Could you check a few things on this model? Use its own coordinates, in mm. Give positions to 0.01 mm unless a question says otherwise; leave off trailing zeros. Order: outer loops, then holes, each group sorted by start corner. A loop starts at its lowest first (then second) coordinate and runs counter-clockwise, first axis right, second up. Notation, with made-up numbers: (33.5, 47) -> (47.5, 47) arc R30 ccw to (47.5, 69) -> close; hole circle Ø5 at (68.25, 62.25). An arc over 180 degrees is marked (long way). Answer as CSV lines item,"result". Start each with the question number.
(1) Will this pin go through, and if not, where does the flat tip stop? pin 1 Ø1.5 at (x, z) = (-5.5, 0.5) entering from -Y.
(2) I want a section at C-C (x = 10.5). Please give me the cut outline in (y, z), plus the area to 3 significant figures.
(3) We'd pull the mould along Y, two halves only. Please class faces 1 (the face through (11.594, 2.281, 1.521)), 2 (the face through (2, 29, 3)), 3 (the face through (10.066, 26.548, 1.479)), 4 (the face through (11.719, 54.594, 1.521)): released by +Y, released by -Y, zero draft, split by the parting line, or undercut.
(4) I want a section at A-A (y = 28.5). Please give me the cut outline in (x, z), plus the area to 3 significant figures.
(5) I need wall thicknesses on L1, parallel to X at y = 28.5, z = 2.3; L2, parallel to Y at x = 10.5, z = 1.6; L3, parallel to Y at x = 9.5, z = 2.75. Which ranges of each line are inside material? Lowest first, please.
(6) I want a section at B-B (z = 1.05). Please give me the cut outline in (x, y).
(7) I want a section at D-D (y = 4.5). Please give me the cut outline in (x, z).
```python
from build123d import *

# Parameters (mm, degrees)
CYLINDER002_R     = 2
CYLINDER002_DEPTH = 10
BOX005_W          = 24
BOX005_H          = 57
BOX005_DEPTH      = 3
FILLET_R          = 8


with BuildPart() as central_bottom_hole:
    # Cylinder002 → Cylinder002 (new body)
    with BuildSketch(Plane(origin=(10.5, 28.5, -4), x_dir=(1, 0, 0), z_dir=(0, 0, 1))):
        Circle(CYLINDER002_R)
    extrude(amount=CYLINDER002_DEPTH)


with BuildPart() as bottom_cut:
    # Box005 → Box005 (new body)
    with BuildSketch(Plane(origin=(-10, 0, 0), x_dir=(1, 0, 0), z_dir=(0, 0, 1))):
        with Locations((12, 28.5)):
            Rectangle(BOX005_W, BOX005_H)
    extrude(amount=BOX005_DEPTH)

    # Fillet
    fillet_edges = [bottom_cut.edges().sort_by_distance(p)[0] for p in [
        (-10, 0, 1.5),
        (-10, 57, 1.5),
        (14, 0, 1.5),
        (14, 57, 1.5),
    ]]
    fillet(fillet_edges, radius=FILLET_R)

    # Cut003: cut central bottom hole
    add(central_bottom_hole.part, mode=Mode.SUBTRACT)


solid = bottom_cut.part
```
Final values:
1,pin 1,"y = 0.49"
2,outline,"(1.39, 0) -> (26.5, 0) -> (26.5, 3) -> (1.39, 3) -> close; (30.5, 0) -> (55.61, 0) -> (55.61, 3) -> (30.5, 3) -> close"
2,area,"151 mm²"
3,face 1,"released by -Y"
3,face 2,"zero draft"
3,face 3,"undercut"
3,face 4,"released by +Y"
4,outline,"(-10, 0) -> (8.5, 0) -> (8.5, 3) -> (-10, 3) -> close; (12.5, 0) -> (14, 0) -> (14, 3) -> (12.5, 3) -> close"
4,area,"60.0 mm²"
5,L1,"-10 to 8.5, 12.5 to 14"
5,L2,"1.39 to 26.5, 30.5 to 55.61"
5,L3,"0.81 to 26.77, 30.23 to 56.19"
6,outline,"(-10, 8) arc R8 ccw to (-2, 0) -> (6, 0) arc R8 ccw to (14, 8) -> (14, 49) arc R8 ccw to (6, 57) -> (-2, 57) arc R8 ccw to (-10, 49) -> close; hole circle Ø4 at (10.5, 28.5)"
7,outline,"(-9.19, 0) -> (13.19, 0) -> (13.19, 3) -> (-9.19, 3) -> close"
